from build123d import *

# Parameters (mm, degrees)
SKETCH1_W           = 152
SKETCH1_H           = 95
BOSS_EXTRUDE2_DEPTH = 92
SKETCH3_W           = 142
SKETCH3_H           = 85
CUT_EXTRUDE2_DEPTH  = 86
SKETCH5_R           = 7.6
SKETCH5_R_2         = 3.6
BOSS_EXTRUDE7_DEPTH = 25.4
SKETCH8_R           = 3.6
CUT_EXTRUDE3_DEPTH  = 202.477045839
SKETCH10_R          = 5
CUT_EXTRUDE7_DEPTH  = 202.477045839
SKETCH13_W          = 115.430222659
SKETCH13_H          = 10.493656606
CUT_EXTRUDE8_DEPTH  = 10


with BuildPart() as part:
    # Sketch1 → Boss-Extrude2 (new body)
    with BuildSketch(Plane(origin=(0, 0, 0), x_dir=(1, 0, 0), z_dir=(0, 1, 0))):
        with Locations((76, 47.5)):
            Rectangle(SKETCH1_W, SKETCH1_H)
    extrude(amount=BOSS_EXTRUDE2_DEPTH)

    # Sketch3 → Cut-Extrude2 (cut)
    with BuildSketch(Plane(origin=(0, 92, 0), x_dir=(1, 0, 0), z_dir=(0, 1, 0))):
        with Locations((76, 47.5)):
            Rectangle(SKETCH3_W, SKETCH3_H)
    extrude(amount=-CUT_EXTRUDE2_DEPTH, mode=Mode.SUBTRACT)

    # Sketch5 → Boss-Extrude7 (add)
    # profile 1 of 4: a face of its own
    with BuildSketch(Plane(origin=(0, 6, 0), x_dir=(1, 0, 0), z_dir=(0, 1, 0))):
        with Locations(Location((20.845338855, 18.593594881, 0), (0, 0, 270))):
            Circle(SKETCH5_R)
        with Locations(Location((20.845338855, 18.593594881, 0), (0, 0, 270))):
            Circle(SKETCH5_R_2, mode=Mode.SUBTRACT)
    # profile 2 of 4: a face of its own
    with BuildSketch(Plane(origin=(0, 6, 0), x_dir=(1, 0, 0), z_dir=(0, 1, 0))):
        with Locations(Location((21.099338855, 74.727594881, 0), (0, 0, 270))):
            Circle(SKETCH5_R)
        with Locations(Location((21.099338855, 74.727594881, 0), (0, 0, 270))):
            Circle(SKETCH5_R_2, mode=Mode.SUBTRACT)
    # profile 3 of 4: a face of its own
    with BuildSketch(Plane(origin=(0, 6, 0), x_dir=(1, 0, 0), z_dir=(0, 1, 0))):
        with Locations(Location((129.303338855, 17.069594881, 0), (0, 0, 270))):
            Circle(SKETCH5_R)
        with Locations(Location((129.303338855, 17.069594881, 0), (0, 0, 270))):
            Circle(SKETCH5_R_2, mode=Mode.SUBTRACT)
    # profile 4 of 4: a face of its own
    with BuildSketch(Plane(origin=(0, 6, 0), x_dir=(1, 0, 0), z_dir=(0, 1, 0))):
        with Locations(Location((129.049338855, 75.235594881, 0), (0, 0, 270))):
            Circle(SKETCH5_R)
        with Locations(Location((129.049338855, 75.235594881, 0), (0, 0, 270))):
            Circle(SKETCH5_R_2, mode=Mode.SUBTRACT)
    extrude(amount=BOSS_EXTRUDE7_DEPTH)

    # Sketch8 → Cut-Extrude3 (cut, through all)
    with BuildSketch(Plane.XY):
        with Locations((20, 77)):
            Circle(SKETCH8_R)
        with Locations((132, 77)):
            Circle(SKETCH8_R)
    extrude(amount=-CUT_EXTRUDE3_DEPTH, mode=Mode.SUBTRACT)

    # Sketch10 → Cut-Extrude7 (cut, through all)
    with BuildSketch(Plane.XZ):
        with Locations(Location((35.489604733, -46.401826634, 0), (0, 0, 270))):
            Circle(SKETCH10_R)
        with Locations(Location((115.489604737, -46.401826637, 0), (0, 0, 270))):
            Circle(SKETCH10_R)
    extrude(amount=-CUT_EXTRUDE7_DEPTH, mode=Mode.SUBTRACT)

    # Sketch13 → Cut-Extrude8 (cut)
    with BuildSketch(Plane(origin=(0, 0, -95), x_dir=(-1, 0, 0), z_dir=(0, 0, -1))):
        with Locations((-76.122019263, 55.234418237)):
            Rectangle(SKETCH13_W, SKETCH13_H)
    extrude(amount=-CUT_EXTRUDE8_DEPTH, mode=Mode.SUBTRACT)


solid = part.part
Could you check a few things on this model? Use its own coordinates, in mm. A direction names the side the tool comes from. Coordinates: 2 decimals unless noted, no trailing zeros. Write each loop counter-clockwise with the first axis right and the second up, starting at its lowest first coordinate (ties: lowest second). Pieces come first, ordered by that corner, then holes. Notation, with made-up numbers: M 10,-16 L 50,-16 A28 ccw 50,3 Z; hole C 10.5,-15.75 d2. An arc over 180 degrees is marked long. One line per question, with ' | ' between items.
1) Imagine slicing it at B-B, the plane y = 14. Give the number of separate pieces and of enclosed holes in the cut face, and give its area (3 significant figures).
Checks:
separate pieces: 5 | enclosed holes: 5 | area: 2,930 mm²
2) Imagine slicing it at D-D, the plane x = 141.5. Write out the boundary of the cut face in (y, z), and give its area (3 significant figures).
Checks:
outline: M 0,-95 L 92,-95 L 92,-90 L 6,-90 L 6,-5 L 92,-5 L 92,0 L 0,0 Z | area: 1,430 mm²
3) For faces 1 (the face through (70, 92, -2)), 2 (the face through (21, 6, -19)), 3 (the face through (18.407, 55, -93)), which set-ups out of +Z, -Z, +X, -X, +Y, -Y let a thin tool reach every point of the face, with its end or its side?
Checks:
face 1: +Z, -Z, +X, -X, +Y | face 2: +Y | face 3: -Z
4) If we mould it in two halves opening along Z, with no side actions, what happens to faces 4 (the face through (136.585, 18.522, -76.225)), 5 (the face through (77, 49.988, -93))? For each: released by +Z, released by -Z, zero draft, split by the parting line, or undercut.
Checks:
face 4: undercut | face 5: zero draft
5) I need wall thicknesses on probe 1 along Y at (x, z) = (132, -93.2); probe 2 along X at (y, z) = (18.5, -41); probe 3 along Z at (x, y) = (133, 66). Which ranges of each line are inside material? Lowest first, please. Write a range as [from, to].
Checks:
probe 1: [0, 49.99], [60.48, 73.4], [80.6, 92] | probe 2: [0, 5], [147, 152] | probe 3: [-95, -90], [-5, 0]
6) Imagine slicing it at C-C, the plane y = 77. Write out the boundary of the cut face in (x, z).
Checks:
outline: M 0,-95 L 16.4,-95 L 16.4,-90 L 5,-90 L 5,-5 L 16.4,-5 L 16.4,0 L 0,0 Z; M 23.6,-95 L 128.4,-95 L 128.4,-90 L 23.6,-90 Z; M 23.6,-5 L 128.4,-5 L 128.4,0 L 23.6,0 Z; M 135.6,-95 L 152,-95 L 152,0 L 135.6,0 L 135.6,-5 L 147,-5 L 147,-90 L 135.6,-90 Z
7) Imagine slicing it at A-A, the plane x = 43. Write out the boundary of the cut face in (y, z).
Checks:
outline: M 0,-95 L 49.99,-95 L 49.99,-90 L 6,-90 L 6,-5 L 92,-5 L 92,0 L 0,0 Z; M 60.48,-95 L 92,-95 L 92,-90 L 60.48,-90 Z
8) For pin 1 Ø12 at (y, z) = (28, -53) entering from -X; pin 2 Ø8 at (x, z) = (38.5, -52.5) entering from +Y; pin 3 Ø3 at (x, y) = (64, 57.5) entering from -Z; pin 4 Ø16.5 at (x, z) = (132.5, -18.5) entering from +Y, each with a flat end and sliding along its axis, tell me the tip position at first contact or that it passes through.
Checks:
pin 1: x = 0 | pin 2: y = 6 | pin 3: z = -5 | pin 4: y = 31.4
